Part model, mm, in its own coordinate system. Face numbers are marked on the shaded views. A direction names the side the tool comes from. Give positions to 0.01 mm unless a question says otherwise; leave off trailing zeros. Order: outer loops, then holes, each group sorted by start corner. A loop starts at its lowest first (then second) coordinate and runs counter-clockwise, first axis right, second up. Notation, with made-up numbers: M -5,-21 L 17,-21 A17 ccw 17,8 Z; hole C -26,-8.5 d1. An arc over 180 degrees is marked long. Return JSON: item names as keys, results as strings.
from build123d import *

# Parameters (mm, degrees)
EXTRUDE_1_DEPTH = 42
EXTRUDE_2_DEPTH = 7
EXTRUDE_3_DEPTH = 17.5
SKETCH_4_R      = 19
EXTRUDE_4_DEPTH = 22.5
SKETCH_5_R      = 1.5
EXTRUDE_5_DEPTH = 6.6
SKETCH_6_R      = 19
EXTRUDE_6_DEPTH = 2
SKETCH_7_R      = 5
EXTRUDE_7_DEPTH = 22.5


with BuildPart() as part:
    # 草图1 → 凸台-拉伸1 (new body)
    with BuildSketch(Plane.XY):
        with BuildLine():
            Line((-16, 21), (16, 21))
            ThreePointArc((16, 21), (19.535533906, 19.535533906), (21, 16))
            Line((21, 16), (21, -16))
            ThreePointArc((21, -16), (19.535533906, -19.535533906), (16, -21))
            Line((16, -21), (-16, -21))
            ThreePointArc((-16, -21), (-19.535533906, -19.535533906), (-21, -16))
            Line((-21, -16), (-21, 16))
            ThreePointArc((-21, 16), (-19.535533906, 19.535533906), (-16, 21))
        make_face()
    extrude(amount=EXTRUDE_1_DEPTH)

    # 草图2 → 凸台-拉伸2 (add)
    with BuildSketch(Plane.XY.offset(42)):
        Polygon((18, 21), (-18, 21), (-21, 18), (-21, -18), (-18, -21), (18, -21), (21, -18), (21, 18), align=None)
    extrude(amount=EXTRUDE_2_DEPTH)

    # 草图3 → 凸台-拉伸3 (add)
    with BuildSketch(Plane.XY.offset(49)):
        with BuildLine():
            Line((-10, 21), (10, 21))
            ThreePointArc((10, 21), (21, 0), (10, -21))
            Line((10, -21), (-10, -21))
            ThreePointArc((-10, -21), (-21, 0), (-10, 21))
        make_face()
    extrude(amount=EXTRUDE_3_DEPTH)

    # 草图4 → 凸台-拉伸4 (add)
    with BuildSketch(Plane.XY.offset(66.5)):
        with Locations(Location((0, 0, 0), (0, 0, 180))):
            Circle(SKETCH_4_R)
    extrude(amount=EXTRUDE_4_DEPTH)

    # 草图5 → 凸台-拉伸5 (add)
    with BuildSketch(Plane.XY.offset(89)):
        with BuildLine():
            Line((-18, 21), (18, 21))
            ThreePointArc((18, 21), (20.121320344, 20.121320344), (21, 18))
            Line((21, 18), (21, -18))
            ThreePointArc((21, -18), (20.121320344, -20.121320344), (18, -21))
            Line((18, -21), (-18, -21))
            ThreePointArc((-18, -21), (-20.121320344, -20.121320344), (-21, -18))
            Line((-21, -18), (-21, 18))
            ThreePointArc((-21, 18), (-20.121320344, 20.121320344), (-18, 21))
        make_face()
        with Locations((-17, 17)):
            Circle(SKETCH_5_R, mode=Mode.SUBTRACT)
        with Locations((17, 17)):
            Circle(SKETCH_5_R, mode=Mode.SUBTRACT)
        with Locations((17, -17)):
            Circle(SKETCH_5_R, mode=Mode.SUBTRACT)
        with Locations((-17, -17)):
            Circle(SKETCH_5_R, mode=Mode.SUBTRACT)
    extrude(amount=EXTRUDE_5_DEPTH)

    # 草图6 → 凸台-拉伸6 (add)
    with BuildSketch(Plane.XY.offset(95.6)):
        with Locations(Location((0, 0, 0), (0, 0, 180))):
            Circle(SKETCH_6_R)
    extrude(amount=EXTRUDE_6_DEPTH)

    # 草图7 → 凸台-拉伸7 (add)
    with BuildSketch(Plane.XY.offset(97.6)):
        with Locations(Location((0, 0, 0), (0, 0, 180))):
            Circle(SKETCH_7_R)
    extrude(amount=EXTRUDE_7_DEPTH)


solid = part.part
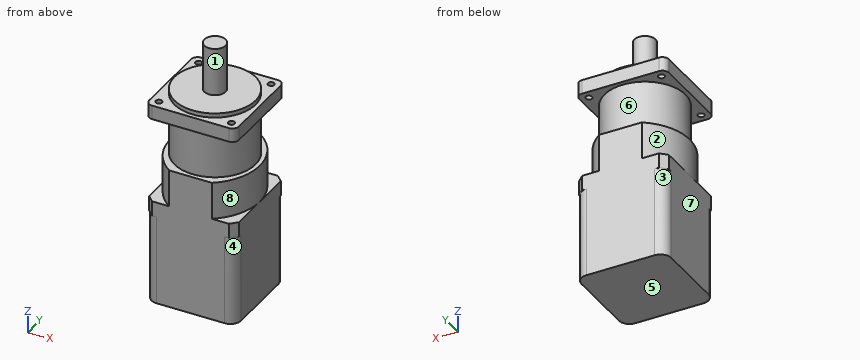
Q1. Band-saw the part on D-D (x = 12). Give the cut face in (y, z), then the cut area to 3 significant figures.
Established:
{"outline": "M -21,0 L 21,0 L 21,49 L 19.46,49 L 19.46,66.5 L 14.73,66.5 L 14.73,89 L 21,89 L 21,95.6 L 14.73,95.6 L 14.73,97.6 L -14.73,97.6 L -14.73,95.6 L -21,95.6 L -21,89 L -14.73,89 L -14.73,66.5 L -19.46,66.5 L -19.46,49 L -21,49 Z", "area": "3,740 mm²"}
Q2. Band-saw the part on A-A (x = -8). Give the cut face in (y, z), then the cut area to 3 significant figures.
Established:
{"outline": "M -21,0 L 21,0 L 21,66.5 L 17.23,66.5 L 17.23,89 L 21,89 L 21,95.6 L 17.23,95.6 L 17.23,97.6 L -17.23,97.6 L -17.23,95.6 L -21,95.6 L -21,89 L -17.23,89 L -17.23,66.5 L -21,66.5 Z", "area": "3,910 mm²"}
Q3. Pin check, flat tips, straight feed: pin 1 (0.8 mm diameter, centred on x = 19.5, y = 19.5, fed in from +Z); pin 2 (2 mm diameter, centred on x = -4, y = 16.5, fed in from +Z); pin 3 (1 mm diameter, centred on y = -4.5, z = 62, fed in from -X). Stop position of each tip, or through.
Established:
{"pin 1": "stops at z = 95.6", "pin 2": "stops at z = 97.6", "pin 3": "stops at x = -20.68"}
Q4. 3-axis set-ups, long thin cutter, end or side, ignore diameter. For the marked faces 1, 2, 3 and 4: which of +Z, -Z, +X, -X, +Y, -Y reach the whole face in a straight line?
Established:
{"face 1": "+Z", "face 2": "-X", "face 3": "-Z, -X, +Y", "face 4": "-Z, +X, -Y"}
Q5. Two-plate mould, pull along Z, no slides. Class the marked faces 5, 6, 7 and 8: +Z half, -Z half, draft (parallel to the pull), parting line (faces both ways), or undercut.
Established:
{"face 5": "-Z half", "face 6": "undercut", "face 7": "draft", "face 8": "undercut"}
Q6. Band-saw the part on B-B (y = 3). Give the cut face in (x, z).
Established:
{"outline": "M -21,0 L 21,0 L 21,49 L 20.82,49 L 20.82,66.5 L 18.76,66.5 L 18.76,89 L 21,89 L 21,95.6 L 18.76,95.6 L 18.76,97.6 L 4,97.6 L 4,120.1 L -4,120.1 L -4,97.6 L -18.76,97.6 L -18.76,95.6 L -21,95.6 L -21,89 L -18.76,89 L -18.76,66.5 L -20.82,66.5 L -20.82,49 L -21,49 Z"}
Q7. Band-saw the part on C-C (z = 81). Give the cut face in (x, y).
Established:
{"outline": "C 0,0 d38"}
Q8. Probe line 1 along Y through (x, z) = (-17, 91); line 2 along Z through (x, y) = (2, 19.5); line 3 along Z through (x, y) = (2, -11.5). List the from-to ranges inside material, lowest first.
Established:
{"line 1": "y = -21 to -18.5, -15.5 to 15.5, 18.5 to 21", "line 2": "z = 0 to 66.5, 89 to 95.6", "line 3": "z = 0 to 97.6"}
